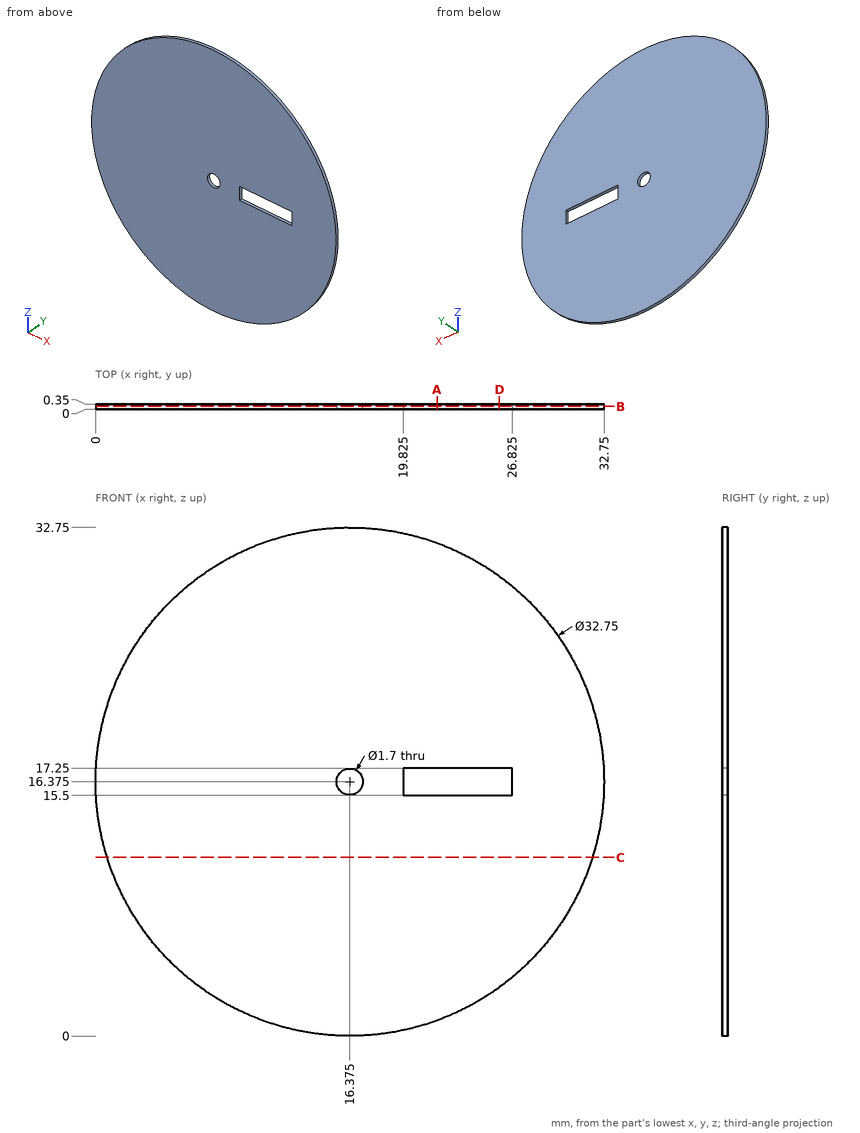
Geometry check sheet. Reference: drawing and pictorial views, mm from the part's lowest x, y, z. Round coordinates to 2 decimals unless told otherwise and drop trailing zeros. Loops run counter-clockwise (first coordinate to the right, second up) from the corner with the lowest first, then second, coordinate; pieces in that order, holes last. Notation, with made-up numbers: (52.5, 6) -> (78.5, 6) arc R17 cw to (78.5, 19) -> close; hole circle Ø11 at (86.5, 71.25). An arc over 180 degrees is marked (long way). Answer as a JSON object with one key per item and string values. Group by question number.
Item 1: Thickness scan on line 1 along X through (y, z) = (0.15, 16.5) (3 decimals); line 2 along Z through (x, y) = (20, 0.2); line 3 along X through (y, z) = (0.05, 16) (3 decimals). Record the ranges inside material, lowest first.
Item 2: Cross-section at B-B, the plane y = 0.2. Record the cut outline in (x, z) (3 decimals).
Item 3: Cross-section at C-C, the plane z = 11.5. Record the cut outline in (x, y), plus the area to 3 significant figures.
Item 4: Cross-section at A-A, the plane x = 22. Record the cut outline in (y, z), plus the area to 3 significant figures.
Item 5: Cross-section at D-D, the plane x = 26. Record the cut outline in (y, z), plus the area to 3 significant figures.
Determined:
{
 "1": {"line 1": "x = 0 to 15.534, 17.216 to 19.825, 26.825 to 32.75", "line 2": "z = 0.41 to 15.5, 17.25 to 32.34", "line 3": "x = 0.004 to 15.612, 17.138 to 19.825, 26.825 to 32.746"},
 "2": {"outline": "circle Ø32.75 at (16.375, 16.375); hole circle Ø1.7 at (16.375, 16.375); hole (19.825, 15.5) -> (26.825, 15.5) -> (26.825, 17.25) -> (19.825, 17.25) -> close"},
 "3": {"outline": "(0.74, 0) -> (32.01, 0) -> (32.01, 0.35) -> (0.74, 0.35) -> close", "area": "10.9 mm²"},
 "4": {"outline": "(0, 1) -> (0.35, 1) -> (0.35, 15.5) -> (0, 15.5) -> close; (0, 17.25) -> (0.35, 17.25) -> (0.35, 31.75) -> (0, 31.75) -> close", "area": "10.2 mm²"},
 "5": {"outline": "(0, 3.13) -> (0.35, 3.13) -> (0.35, 15.5) -> (0, 15.5) -> close; (0, 17.25) -> (0.35, 17.25) -> (0.35, 29.62) -> (0, 29.62) -> close", "area": "8.66 mm²"}
}
